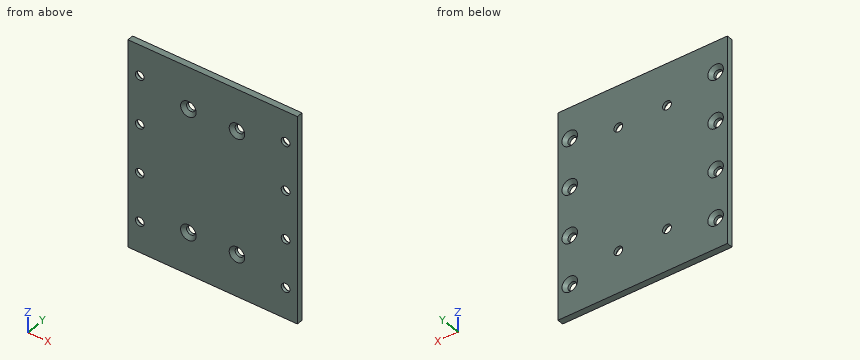
from build123d import *

# Parameters (mm, degrees)
SKETCH2_W                    = 87.12
SKETCH2_H                    = 106.68
BOSS_EXTRUDE1_DEPTH          = 3.175
CSK_FOR_M4_SFHCS1_AT_2_COUNT = 2
CSK_FOR_M4_SFHCS1_AT_2_PITCH = 25


# Read off the part's stored shape, not the designer's step: AdvancedHole2
with BuildPart() as part:
    # Sketch2 → Boss-Extrude1 (new body)
    with BuildSketch(Plane(origin=(0, 0, 0), x_dir=(1, 0, 0), z_dir=(0, 1, 0))):
        Rectangle(SKETCH2_W, SKETCH2_H)
    extrude(amount=BOSS_EXTRUDE1_DEPTH)

    # AdvancedHole2 outline → AdvancedHole2 (revolve, cut)
    with BuildSketch(Plane(origin=(-37.5, 0, 12.5), x_dir=(1, 0, 0), z_dir=(0, 0, 1))):
        Polygon((4, 3.175), (0, 3.175), (0, 0), (2.25, 0), (2.25, 1.425), align=None)
    revolve(axis=Axis((-37.5, 0, 12.5), (0, 1, 0)), mode=Mode.SUBTRACT)

    # AdvancedHole2 2 outline → AdvancedHole2 2 (revolve, cut)
    with BuildSketch(Plane(origin=(-37.5, 0, 37.5), x_dir=(1, 0, 0), z_dir=(0, 0, 1))):
        Polygon((4, 3.175), (0, 3.175), (0, 0), (2.25, 0), (2.25, 1.425), align=None)
    revolve(axis=Axis((-37.5, 0, 37.5), (0, 1, 0)), mode=Mode.SUBTRACT)

    # AdvancedHole2 3 outline → AdvancedHole2 3 (revolve, cut)
    with BuildSketch(Plane(origin=(37.5, 0, 37.5), x_dir=(1, 0, 0), z_dir=(0, 0, 1))):
        Polygon((4, 3.175), (0, 3.175), (0, 0), (2.25, 0), (2.25, 1.425), align=None)
    revolve(axis=Axis((37.5, 0, 37.5), (0, 1, 0)), mode=Mode.SUBTRACT)

    # AdvancedHole2 4 outline → AdvancedHole2 4 (revolve, cut)
    with BuildSketch(Plane(origin=(37.5, 0, 12.5), x_dir=(1, 0, 0), z_dir=(0, 0, 1))):
        Polygon((4, 3.175), (0, 3.175), (0, 0), (2.25, 0), (2.25, 1.425), align=None)
    revolve(axis=Axis((37.5, 0, 12.5), (0, 1, 0)), mode=Mode.SUBTRACT)

    # AdvancedHole2 5 outline → AdvancedHole2 5 (revolve, cut)
    with BuildSketch(Plane(origin=(37.5, 0, -12.5), x_dir=(1, 0, 0), z_dir=(0, 0, 1))):
        Polygon((4, 3.175), (0, 3.175), (0, 0), (2.25, 0), (2.25, 1.425), align=None)
    revolve(axis=Axis((37.5, 0, -12.5), (0, 1, 0)), mode=Mode.SUBTRACT)

    # AdvancedHole2 6 outline → AdvancedHole2 6 (revolve, cut)
    with BuildSketch(Plane(origin=(37.5, 0, -37.5), x_dir=(1, 0, 0), z_dir=(0, 0, 1))):
        Polygon((4, 3.175), (0, 3.175), (0, 0), (2.25, 0), (2.25, 1.425), align=None)
    revolve(axis=Axis((37.5, 0, -37.5), (0, 1, 0)), mode=Mode.SUBTRACT)

    # AdvancedHole2 7 outline → AdvancedHole2 7 (revolve, cut)
    with BuildSketch(Plane(origin=(-37.5, 0, -12.5), x_dir=(1, 0, 0), z_dir=(0, 0, 1))):
        Polygon((4, 3.175), (0, 3.175), (0, 0), (2.25, 0), (2.25, 1.425), align=None)
    revolve(axis=Axis((-37.5, 0, -12.5), (0, 1, 0)), mode=Mode.SUBTRACT)

    # AdvancedHole2 8 outline → AdvancedHole2 8 (revolve, cut)
    with BuildSketch(Plane(origin=(-37.5, 0, -37.5), x_dir=(1, 0, 0), z_dir=(0, 0, 1))):
        Polygon((4, 3.175), (0, 3.175), (0, 0), (2.25, 0), (2.25, 1.425), align=None)
    revolve(axis=Axis((-37.5, 0, -37.5), (0, 1, 0)), mode=Mode.SUBTRACT)

    # Sketch21 → CSK for M4 SFHCS1 (revolve, cut)
    with BuildSketch(Plane(origin=(12.5, 0, -31.75), x_dir=(0, 0, -1), z_dir=(1, 0, 0))):
        Polygon((0, 0), (0, 11.351936393), (2.25, 10), (2.25, 1.75), (4, 0), align=None)
    csk_for_m4_sfhcs1 = revolve(axis=Axis((12.5, -6.35, -31.75), (0, 1, 0)), mode=Mode.SUBTRACT)

    # CSK for M4 SFHCS1 at 2: CSK for M4 SFHCS1 ×2
    with Locations(*[(-i * CSK_FOR_M4_SFHCS1_AT_2_PITCH, 0, 0) for i in range(1, CSK_FOR_M4_SFHCS1_AT_2_COUNT)]):
        add(csk_for_m4_sfhcs1, mode=Mode.SUBTRACT)

    # Mirror1: CSK for M4 SFHCS1 across plane
    add(csk_for_m4_sfhcs1.mirror(Plane.XY), mode=Mode.SUBTRACT)

    # Mirror1 copy 1 sketch → Mirror1 copy 1 (revolve, cut)
    with BuildSketch(Plane(origin=(-12.5, 0, 31.75), x_dir=(0, 0, 1), z_dir=(1, 0, 0))):
        Polygon((0, 0), (0, -11.351936393), (2.25, -10), (2.25, -1.75), (4, 0), align=None)
    revolve(axis=Axis((-12.5, -6.35, 31.75), (0, -1, 0)), mode=Mode.SUBTRACT)


solid = part.part
Input: part model. Units: mm. Frame: model coordinates. Coordinates: 2 decimals unless noted, no trailing zeros. Loops run counter-clockwise (first coordinate to the right, second up) from the corner with the lowest first, then second, coordinate; pieces in that order, holes last. Notation, with made-up numbers: (54.25, 49) - (85.25, 49) arc R10 ccw to (85.25, 60) - close; hole circle Ø11 at (-31, -38). An arc over 180 degrees is marked (long way). Answer in a Markdown table with one row per item. Add a question column.
Item 1: Section query B-B on x = 12.5. Return the cut outline in (y, z) (3 decimals), then the cut area to 3 significant figures.
Item 2: Line query: line 1 along Z through (x, y) = (37.5, 0.65); line 2 along X through (y, z) = (0.6, 12.5); line 3 along Z through (x, y) = (12.5, 2.15). Output: solid intervals per line, ascending. Write a range as [from, to].
Item 3: Section query C-C on x = -37.5. Return the cut outline in (y, z) (3 decimals), then the cut area to 3 significant figures.
Item 4: Section query A-A on z = 37.5. Return the cut outline in (x, y) (3 decimals).
Item 5: Contact query for flat-ended pins moving along their axis: P1, Ø7, axis at x = 37.5, z = 12.5, coming from the +Y side (3 decimals); P2, Ø5, axis at x = 12.5, z = 31.75, coming from the -Y side. Output: stop coordinate, or through.
Recorded:
| question | item | result |
|---|---|---|
| 1 | outline | (0, -53.34) - (3.175, -53.34) - (3.175, -34) - (1.75, -34) - (0, -35.75) - close; (0, -27.75) - (1.75, -29.5) - (3.175, -29.5) - (3.175, 29.5) - (1.75, 29.5) - (0, 27.75) - close; (0, 35.75) - (1.75, 34) - (3.175, 34) - (3.175, 53.34) - (0, 53.34) - close |
| 1 | area | 304 mm^2 |
| 2 | line 1 | [-53.34, -39.75], [-35.25, -14.75], [-10.25, 10.25], [14.75, 35.25], [39.75, 53.34] |
| 2 | line 2 | [-43.56, -39.75], [-35.25, 35.25], [39.75, 43.56] |
| 2 | line 3 | [-53.34, -34], [-29.5, 29.5], [34, 53.34] |
| 3 | outline | (0, -53.34) - (3.175, -53.34) - (3.175, -41.5) - (1.425, -39.75) - (0, -39.75) - close; (0, -35.25) - (1.425, -35.25) - (3.175, -33.5) - (3.175, -16.5) - (1.425, -14.75) - (0, -14.75) - close; (0, -10.25) - (1.425, -10.25) - (3.175, -8.5) - (3.175, 8.5) - (1.425, 10.25) - (0, 10.25) - close; (0, 14.75) - (1.425, 14.75) - (3.175, 16.5) - (3.175, 33.5) - (1.425, 35.25) - (0, 35.25) - close; (0, 39.75) - (1.425, 39.75) - (3.175, 41.5) - (3.175, 53.34) - (0, 53.34) - close |
| 3 | area | 269 mm^2 |
| 4 | outline | (-43.56, 0) - (-39.75, 0) - (-39.75, 1.425) - (-41.5, 3.175) - (-43.56, 3.175) - close; (-35.25, 0) - (35.25, 0) - (35.25, 1.425) - (33.5, 3.175) - (-33.5, 3.175) - (-35.25, 1.425) - close; (39.75, 0) - (43.56, 0) - (43.56, 3.175) - (41.5, 3.175) - (39.75, 1.425) - close |
| 5 | P1 | y = 2.675 |
| 5 | P2 | y = 1.5 |
